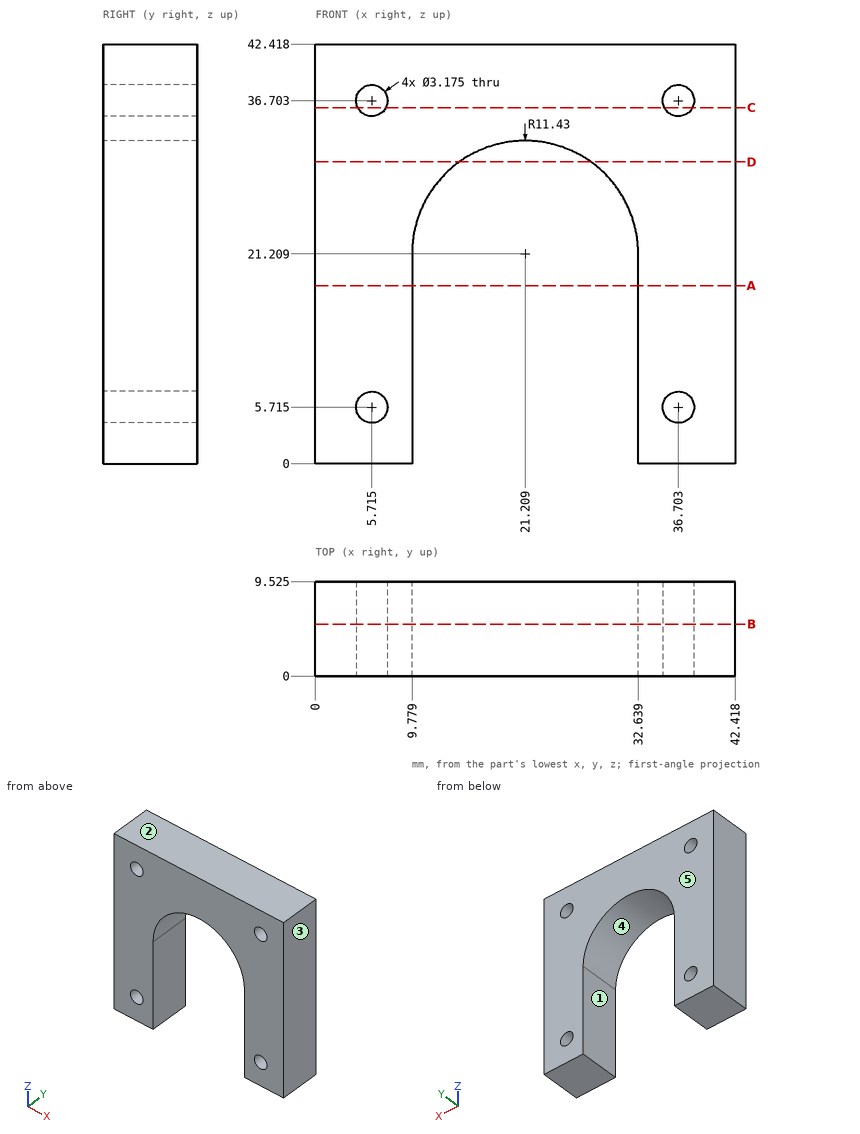
Print and shaded views of the part. All mm, measured from the part's lowest x, y and z. A direction names the side the tool comes from. Coordinates: 2 decimals unless noted, no trailing zeros. Order: outer loops, then holes, each group sorted by start corner. A loop starts at its lowest first (then second) coordinate and runs counter-clockwise, first axis right, second up. Notation, with made-up numbers: (-1, 7) -> (11, 7) arc R29 ccw to (11, 46) -> close; hole circle Ø5 at (-16.5, 35.5). An arc over 180 degrees is marked (long way). Answer as a JSON object with one key per item and string values. Group by question number.
1) Flat gauge pins, fed straight in: pin 1 (2.5 mm diameter, centred on x = 36.703, z = 5.715, fed in from -Y); pin 2 (6 mm diameter, centred on x = 36, z = 11, fed in from -Y); pin 3 (2 mm diameter, centred on x = 21.5, y = 3.5, fed in from -Z). Where does each tip first touch, or does it go through?
2) Drill centre lines: L1, parallel to X at y = 8, z = 14; L2, parallel to Z at x = 5, y = 7; L3, parallel to X at y = 6.5, z = 4.5. Where is each one in solid material? Low to high.
3) Cut at C-C, the plane z = 36. Write the cut outline in (x, y) (3 decimals).
4) Pull direction X, two halves, no side cores. Call the marked faces 3, 4 and 5: +X half, -X half, draft (parallel to the pull), parting line (faces both ways), or undercut.
5) Cut at D-D, the plane z = 30.5. Write the cut outline in (x, y) (1 decimal), then the cut area to 3 significant figures.
6) Cut at B-B, the plane y = 5.25. Write the cut outline in (x, z) (1 decimal), then the cut area to 3 significant figures.
7) Which spindle directions (+Z, -Z, +X, -X, +Y, -Y) get a long thin tool onto all of the face, cutting with end or side? Do the marked faces 1 and 2. Say none if no direction does.
8) Cut at A-A, the plane z = 18. Write the cut outline in (x, y) (3 decimals), then the cut area to 3 significant figures.
Check values:
{
 "1": {"pin 1": "passes through", "pin 2": "stops at y = 0", "pin 3": "stops at z = 32.57"},
 "2": {"L1": "x = 0 to 9.78, 32.64 to 42.42", "L2": "z = 0 to 4.3, 7.13 to 35.29, 38.12 to 42.42", "L3": "x = 0 to 4.69, 6.74 to 9.78, 32.64 to 35.68, 37.72 to 42.42"},
 "3": {"outline": "(0, 0) -> (4.292, 0) -> (4.292, 9.525) -> (0, 9.525) -> close; (7.138, 0) -> (35.28, 0) -> (35.28, 9.525) -> (7.138, 9.525) -> close; (38.126, 0) -> (42.418, 0) -> (42.418, 9.525) -> (38.126, 9.525) -> close"},
 "4": {"face 3": "+X half", "face 4": "undercut", "face 5": "draft"},
 "5": {"outline": "(0, 0) -> (14.6, 0) -> (14.6, 9.5) -> (0, 9.5) -> close; (27.9, 0) -> (42.4, 0) -> (42.4, 9.5) -> (27.9, 9.5) -> close", "area": "277 mm²"},
 "6": {"outline": "(0, 0) -> (9.8, 0) -> (9.8, 21.2) arc R11.4 cw to (32.6, 21.2) -> (32.6, 0) -> (42.4, 0) -> (42.4, 42.4) -> (0, 42.4) -> close; hole circle Ø3.2 at (5.7, 5.7); hole circle Ø3.2 at (5.7, 36.7); hole circle Ø3.2 at (36.7, 5.7); hole circle Ø3.2 at (36.7, 36.7)", "area": "1,080 mm²"},
 "7": {"face 1": "-Z, +Y, -Y", "face 2": "+Z, +X, -X, +Y, -Y"},
 "8": {"outline": "(0, 0) -> (9.779, 0) -> (9.779, 9.525) -> (0, 9.525) -> close; (32.639, 0) -> (42.418, 0) -> (42.418, 9.525) -> (32.639, 9.525) -> close", "area": "186 mm²"}
}
